from build123d import *

# Parameters (mm, degrees)
F0_R     = 1.45
F1_DEPTH = 10
F2_R     = 2.9
F3_DEPTH = 2.4
F4_R     = 1
F5_W     = 1
F5_H     = 1
F6_DEPTH = 1.5


with BuildPart() as f1:
    # F0 (on Top) → F1 (new body)
    with BuildSketch(Plane.XY):
        Circle(F0_R)
    extrude(amount=F1_DEPTH)

    # F2 (on Top) → F3 (join)
    with BuildSketch(Plane.XY):
        Circle(F2_R)
    extrude(amount=-F3_DEPTH)

    # F4
    f4_edges = [f1.edges().sort_by_distance(p)[0] for p in [
        (-2.9, 0, -2.4),
    ]]
    fillet(f4_edges, radius=F4_R)

    # F5 (on face) → F6 (cut)
    with BuildSketch(Plane(origin=(0, 0, -2.4), x_dir=(1, 0, 0), z_dir=(0, 0, -1))):
        with Locations((1, 0)):
            Rectangle(F5_W, F5_H)
        Rectangle(F5_W, F5_H)
        with Locations((0, 1)):
            Rectangle(F5_W, F5_H)
        with Locations((-1, 0)):
            Rectangle(F5_W, F5_H)
        with Locations((0, -1)):
            Rectangle(F5_W, F5_H)
    extrude(amount=-F6_DEPTH, mode=Mode.SUBTRACT)


solid = f1.part
Geometry check sheet. Reference: the model listing, model coordinates, mm. A direction names the side the tool comes from. Round coordinates to 2 decimals unless told otherwise and drop trailing zeros. Write each loop counter-clockwise with the first axis right and the second up, starting at its lowest first coordinate (ties: lowest second). Pieces come first, ordered by that corner, then holes.
Item 1: Go/stop test with flat-tipped pins: pin 1 Ø0.8 at (y, z) = (1, -1.5) entering from +X; pin 2 Ø0.5 at (x, z) = (-1, -2) entering from -Y; pin 3 Ø3 at (x, z) = (-1, 5.5) entering from -Y. Record where each tip stops, or that it passes through.
Determined:
pin 1: stops at x = 2.84
pin 2: stops at y = -2.69
pin 3: stops at y = -1.45
Item 2: Section check C-C (z = 8.5). Record the boundary of the cut face in (x, y), plus the area to 3 significant figures.
Determined:
outline: circle Ø2.9 at (0, 0)
area: 6.61 mm2
Item 3: Mould release check, pull along Y, two halves, no side actions. Record for faces 4 (the face through (1, -1, -2.4)), 5 (the face through (-2.9, 0.1, -0.7)), 6 (the face through (1, -0.5, -2)): +Y half, -Y half, draft (parallel to the pull), parting line (faces both ways), or undercut.
Determined:
face 4: draft
face 5: parting line
face 6: undercut
Item 4: Section check D-D (z = -0.25). Record the boundary of the cut face in (x, y).
Determined:
outline: circle Ø5.8 at (0, 0)
Item 5: Section check A-A (y = 0). Record the boundary of the cut face in (x, z), plus the area to 3 significant figures.
Determined:
outline: (-2.9, -1.4) arc R1 ccw to (-1.9, -2.4) - (-1.5, -2.4) - (-1.5, -0.9) - (1.5, -0.9) - (1.5, -2.4) - (1.9, -2.4) arc R1 ccw to (2.9, -1.4) - (2.9, 0) - (1.45, 0) - (1.45, 10) - (-1.45, 10) - (-1.45, 0) - (-2.9, 0) - close
area: 38.0 mm2
Item 6: Material ranges on line 1 along Z through (x, y) = (0.25, -0.8); line 2 along Z through (x, y) = (-0.9, -1.75); line 3 along X through (y, z) = (1.6, -0.5), recorded low to high.
Determined:
line 1: z = -0.9 to 10
line 2: z = -2.4 to 0
line 3: x = -2.42 to 2.42
Item 7: Access from +Z, -Z, +X, -X, +Y, -Y to the whole of each face (thin tool, end or side, straight path). Record for faces 1 (the face through (1.5, 0, -2)), 2 (the face through (0, 0, 10)), 3 (the face through (1.2, -1.2, 0)).
Determined:
face 1: -Z
face 2: +Z, +X, -X, +Y, -Y
face 3: +Z
